Autodesk Inventor part; units mm, degrees
ref_plane "YZ Plane" through (0, 0, 0) normal (1, 0, 0) x (0, 1, 0)
ref_plane "XZ Plane" through (0, 0, 0) normal (0, 1, 0) x (-1, 0, 0)
ref_plane "XY Plane" through (0, 0, 0) normal (0, 0, 1) x (1, 0, 0)
sketch "スケッチ1" plane through (0, 0, 0) normal (0, 1, 0) x (-1, 0, 0)
  line L0 (0, 0) -> (-230, 0)
  line L1 (-230, 0) -> (-230, -35)
  line L2 (-230, -35) -> (0, -35)
  line L3 (0, -35) -> (0, 0)
  arc A0 (0, -35) -> (0, 0) centre (0, -17.5) ccw
  dimension "d0" = 230
  dimension "d1" = 35
  dimension "d2" = 17.5
extrude "押し出し1" add sketch "スケッチ1" along normal blind 3
sketch "スケッチ2" plane through (0, 3, 0) normal (0, 1, 0) x (1, 0, 0)
  line L0 (0, 17.5) -> (238.6526, 17.5)
  line L1 (0, 0) -> (230, 0)
  arc A0 (0, 35) -> (0, 0) centre (0, 17.5) ccw
  point P0 (90, 17.5)
  point P1 (100, 17.5)
  point P2 (110, 17.5)
  point P3 (120, 17.5)
  point P4 (130, 17.5)
  point P5 (140, 17.5)
  point P6 (150, 17.5)
  point P7 (160, 17.5)
  point P8 (170, 17.5)
  point P9 (180, 17.5)
  point P10 (190, 17.5)
  point P11 (200, 17.5)
  point P12 (210, 17.5)
  point P13 (-17.5, 17.5)
  point P14 (220, 17.5)
  point P15 (80, 17.5)
  point P16 (32, 17.5)
  point P17 (22, 17.5)
  dimension "d5" = 17.5
  dimension "d13" = 10
  dimension "d14" = 10
  dimension "d15" = 10
  dimension "d16" = 10
  dimension "d17" = 10
  dimension "d18" = 10
  dimension "d19" = 10
  dimension "d20" = 10
  dimension "d21" = 10
  dimension "d22" = 10
  dimension "d23" = 10
  dimension "d24" = 10
  dimension "d35" = 17.5
  dimension "d67" = 10
  dimension "d78" = 10
  dimension "d81" = 10
  dimension "d82" = 48
hole "穴1" at (90, 3, -17.5) at (100, 3, -17.5) at (110, 3, -17.5) at (120, 3, -17.5) at (130, 3, -17.5) at (140, 3, -17.5) at (150, 3, -17.5) at (160, 3, -17.5) at (170, 3, -17.5) at (180, 3, -17.5) at (190, 3, -17.5) at (200, 3, -17.5) at (210, 3, -17.5) at (220, 3, -17.5) at (80, 3, -17.5) at (32, 3, -17.5) at (22, 3, -17.5) direction (0, -1, 0) diameter 3.2 end through all
sketch "スケッチ3" plane through (0, 3, 0) normal (0, 1, 0) x (1, 0, 0)
  line L0 (230, 35) -> (0, 35)
  point P0 (0, 0)
  point P1 (0, 17.5)
  dimension "d36" = 17.5
hole "穴2" at (0, 3, -17.5) direction (0, -1, 0) diameter 16 end through all
sketch "スケッチ4" plane through (0, 3, 0) normal (0, 1, 0) x (1, 0, 0)
  circle A0 centre (0, 17.5) radius 6
  circle A1 centre (0, 17.5) radius 8
  line L0 (-0.1439, 17.5) -> (-6.5454, 17.5)
  line L1 (-6.5454, 17.5) -> (7.5104, 17.5)
  point P0 (0, 0)
  point P1 (0, 11.5)
  point P2 (6, 17.5)
  point P3 (0, 23.5)
  point P4 (-6, 17.5)
  dimension "d44" = 12
  dimension "d45" = 0
hole "穴3" [suppressed]
sketch "スケッチ5" plane through (0, 3, 0) normal (0, 1, 0) x (1, 0, 0)
  circle A0 centre (0, 17.5) radius 8
  point P0 (0, 0)
  point P1 (15.8, 7)
  point P2 (15.8, 28)
  point P3 (24.9999, 17.5)
  dimension "d53" = 10.5
  dimension "d55" = 15.8
  dimension "d56" = 15.8
  dimension "d83" = 10.5
hole "穴4" [suppressed]
sketch "スケッチ6" plane through (0, 3, 0) normal (0, 1, 0) x (1, 0, 0)
  circle A0 centre (0, 17.5) radius 8 construction
  line L0 (0, 17.5) -> (230, 17.5) construction
  line L1 (230, 0) -> (230, 35) construction
  point P0 (0, 0)
  point P1 (67, 17.5)
  point P2 (47, 17.5)
  dimension "d69" = 47
  dimension "d70" = 20
hole "穴5" at (67, 3, -17.5) at (47, 3, -17.5) direction (0, -1, 0) diameter 6.4 end through all
sketch "スケッチ7" plane through (0, 3, 0) normal (0, 1, 0) x (1, 0, 0)
  circle A0 centre (0, 17.5) radius 8 construction
  circle A1 centre (0, 17.5) radius 12.5 construction
  point P0 (0, 0)
  point P1 (0, 5)
  point P2 (12.5, 17.5)
  point P3 (0, 30)
  point P4 (-12.5, 17.5)
  dimension "d84" = 25
  dimension "d87" = 360
hole "穴6" at (0, 3, -5) at (12.5, 3, -17.5) at (0, 3, -30) at (-12.5, 3, -17.5) direction (0, -1, 0) diameter 3.2 end through all
properties part number "arm_plate" material "アルミニウム 5052"
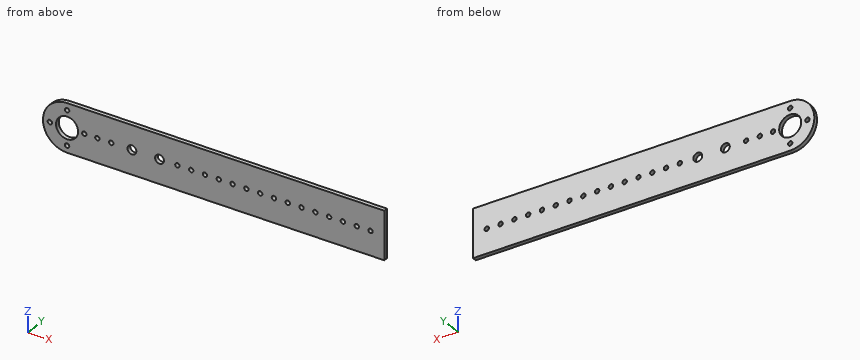
Input: part model. Units: mm. Frame: model coordinates. Coordinates: 2 decimals unless noted, no trailing zeros. Write each question's results on one line, items separated by ' | '.
Item 1: Section query A-A on y = 0.8. Count the separate pieces of the cut face and the enclosed holes in it, plus the area to 3 significant figures.
Conclusion:
separate pieces: 1 | enclosed holes: 24 | area: 8,100 mm^2
Item 2: Pin query (flat end, axial travel): pin 1 Ø2.5 at (x, z) = (120, -17.5) entering from -Y. Return the tip coordinate at first contact, or that it passes through.
Conclusion:
pin 1: passes through
Item 3: Material intervals for probe 1 along Z at (x, y) = (0, 1.8); probe 2 along Z at (x, y) = (90, 0.9); probe 3 along Z at (x, y) = (220.5, 0.3), sorted ascending.
Conclusion:
probe 1: z = -35 to -31.6, -28.4 to -25.5, -9.5 to -6.6, -3.4 to 0 | probe 2: z = -35 to -19.1, -15.9 to 0 | probe 3: z = -35 to -19.02, -15.98 to 0
